Autodesk Inventor part; units mm, degrees
ref_plane "YZ Plane" through (0, 0, 0) normal (1, 0, 0) x (0, 1, 0)
ref_plane "XZ Plane" through (0, 0, 0) normal (0, 1, 0) x (-1, 0, 0)
ref_plane "XY Plane" through (0, 0, 0) normal (0, 0, 1) x (1, 0, 0)
sketch "Sketch1" plane through (0, 0, 0) normal (0, 0, 1) x (1, 0, 0)
  line L0 (-5.3, 7.3) -> (5.3, 7.3)
  line L1 (7.3, 5.3) -> (7.3, -5.3)
  line L2 (5.3, -7.3) -> (-5.3, -7.3)
  line L3 (-7.3, -5.3) -> (-7.3, 5.3)
  arc A0 (-5.3, 7.3) -> (-7.3, 5.3) centre (-5.3, 5.3) ccw
  arc A1 (7.3, 5.3) -> (5.3, 7.3) centre (5.3, 5.3) ccw
  arc A2 (5.3, -7.3) -> (7.3, -5.3) centre (5.3, -5.3) ccw
  arc A3 (-7.3, -5.3) -> (-5.3, -7.3) centre (-5.3, -5.3) ccw
  line L4 (-7.3, 4) -> (-10, 4)
  line L5 (-10, 4) -> (-10, 3)
  line L6 (-10, 3) -> (-11, 3)
  line L7 (-11, 3) -> (-11, 4)
  line L8 (-11, 4) -> (-13, 4)
  line L9 (-13, 4) -> (-13, 0)
  line L10 (-13, 0) -> (-7.3, 0)
  circle A4 centre (0, 0) radius 3
  point P0 (0, 7.3)
  point P1 (7.3, 0)
  dimension "d0" = 14.6
  dimension "d1" = 2
  dimension "d3" = 8
  dimension "d4" = 6
  dimension "d5" = 2
  dimension "d6" = 1
  dimension "d7" = 13
  dimension "d11" = 6
extrude "Extrusion1" add sketch "Sketch1" along normal mid plane 15 contours L0 A1 L1 A2 L2 A3 L3 A0
revolve "Revolution1" add sketch "Sketch1" angle 360 about axis through (-13, 0, 0) along (1, 0, 0) contours L3 L10 L9 L8 L7 L6 L5 L4
mirror "Mirror1" about plane through (0, 0, 0) normal (1, 0, 0) of "Revolution1"
chamfer "Chamfer1" distance 0.5 angle 45 4 edges at (13, -4, 0) (-13, -4, 0) (-3, 0, 7.5) (-3, 0, -7.5)
properties part number "Tee" material "Steel, Mild"
Check sheet for the modelled part. Datum: model origin and axes. Units: mm. A direction names the side the tool comes from. Round coordinates to 2 decimals unless told otherwise and drop trailing zeros. Order: outer loops, then holes, each group sorted by start corner. A loop starts at its lowest first (then second) coordinate and runs counter-clockwise, first axis right, second up. Notation, with made-up numbers: (14.25, 53.5) -> (33.25, 53.5) arc R19 ccw to (33.25, 59.5) -> close; hole circle Ø3 at (40, -18). An arc over 180 degrees is marked (long way). One line per item, written item: value. Start each with the question number.
Q1. Thickness scan on line 1 (Y direction, x = 0, z = 4); line 2 (X direction, y = 1.75, z = 0); line 3 (X direction, y = 2, z = -4.5). Record the ranges inside material, lowest first.
Q2. Cross-section at A-A (x = 0). Record the boundary of the cut face in (y, z).
Q3. Cross-section at B-B (z = 5.75). Record the boundary of the cut face in (x, y).
Q4. Set-up check for faces 1 (the face through (11.76, -0.867, -3.905)), 2 (the face through (-11, 1, 3)), 3 (the face through (6.7, 6.73, -0.11)), 4 (the face through (6.73, -6.7, -0.11)), 5 (the face through (-11.76, -0.867, 3.905)): record each of +Z, -Z, +X, -X, +Y, -Y from which the full face is reachable in a straight line by a thin tool's end or side.
Q5. Gauge pin test, flat ends, axial feed: pin 1 Ø1.5 at (y, z) = (-4, 5) entering from +X; pin 2 Ø5.5 at (x, y) = (0, 0) entering from -Z. Record the tip position at first contact, or that the pin passes through.
Q6. Cross-section at D-D (x = -6.25). Record the boundary of the cut face in (y, z), and give its area (3 significant figures).
Q7. Cross-section at C-C (x = 10.5). Record the boundary of the cut face in (y, z), and give its area (3 significant figures).
Completed:
1. line 1: y = -7.3 to -3, 3 to 7.3
1. line 2: x = -13 to -2.44, 2.44 to 13
1. line 3: x = -7.3 to -2.24, 2.24 to 7.3
2. outline: (-7.3, -7.5) -> (-3.5, -7.5) -> (-3, -7) -> (-3, 7) -> (-3.5, 7.5) -> (-7.3, 7.5) -> close; (3, -7) -> (3.5, -7.5) -> (7.3, -7.5) -> (7.3, 7.5) -> (3.5, 7.5) -> (3, 7) -> close
3. outline: (-7.3, -5.3) arc R2 ccw to (-5.3, -7.3) -> (5.3, -7.3) arc R2 ccw to (7.3, -5.3) -> (7.3, 5.3) arc R2 ccw to (5.3, 7.3) -> (-5.3, 7.3) arc R2 ccw to (-7.3, 5.3) -> close; hole circle Ø6 at (0, 0)
4. face 1: +X
4. face 2: none
4. face 3: +Z, -Z, +X, +Y
4. face 4: +Z, -Z, +X, -Y
4. face 5: -X
5. pin 1: stops at x = 7.3
5. pin 2: passes through
6. outline: (-7.06, -7.5) -> (7.06, -7.5) -> (7.06, 7.5) -> (-7.06, 7.5) -> close
6. area: 212 mm²
7. outline: circle Ø6 at (0, 0)
7. area: 28.3 mm²
